Model file for the job. Use its own axes, mm. A direction names the side the tool comes from. Give positions to 0.01 mm unless a question says otherwise; leave off trailing zeros. Write each loop counter-clockwise with the first axis right and the second up, starting at its lowest first coordinate (ties: lowest second). Pieces come first, ordered by that corner, then holes.
```python
from build123d import *

# Parameters (mm, degrees)
SKIZZE1_R                       = 12.4
AUFSATZ_LINEAR_AUSTRAGEN1_DEPTH = 38.8
SKIZZE2_R                       = 3.75
AUFSATZ_LINEAR_AUSTRAGEN2_DEPTH = 2
SKIZZE3_R                       = 2
AUFSATZ_LINEAR_AUSTRAGEN3_DEPTH = 10
SKIZZE4_W                       = 7
SKIZZE4_H                       = 2
AUFSATZ_LINEAR_AUSTRAGEN4_DEPTH = 3


with BuildPart() as part:
    # Skizze1 → Aufsatz-Linear austragen1 (new body)
    with BuildSketch(Plane.XY):
        Circle(SKIZZE1_R)
    extrude(amount=AUFSATZ_LINEAR_AUSTRAGEN1_DEPTH)

    # Skizze2 → Aufsatz-Linear austragen2 (add)
    with BuildSketch(Plane.XY.offset(38.8)):
        Circle(SKIZZE2_R)
    extrude(amount=AUFSATZ_LINEAR_AUSTRAGEN2_DEPTH)

    # Skizze3 → Aufsatz-Linear austragen3 (add)
    with BuildSketch(Plane.XY.offset(40.8)):
        Circle(SKIZZE3_R)
    extrude(amount=AUFSATZ_LINEAR_AUSTRAGEN3_DEPTH)

    # Skizze4 → Aufsatz-Linear austragen4 (add)
    with BuildSketch(Plane(origin=(0, 0, 0), x_dir=(-1, 0, 0), z_dir=(0, 0, -1))):
        with Locations((0, -9)):
            Rectangle(SKIZZE4_W, SKIZZE4_H)
    extrude(amount=AUFSATZ_LINEAR_AUSTRAGEN4_DEPTH)


solid = part.part
```
1. Probe probe 1 along Z at (x, y) = (1.5, -10.5); probe 2 along Z at (x, y) = (-1.5, -2); probe 3 along X at (y, z) = (-0.25, 19). List the from-to ranges inside material, lowest first.
Calculated:
probe 1: z = 0 to 38.8
probe 2: z = 0 to 40.8
probe 3: x = -12.4 to 12.4
2. Pull direction Y, two halves, no side cores. Call faces 1 (the flat face through (0, -9, -3)), 2 (the flat face through (0, -8, -1)), 3 (the flat face through (0, -10, -1)), 4 (the cylindrical face through (0, -2, 46)): +Y half, -Y half, draft (parallel to the pull), parting line (faces both ways), or undercut.
Calculated:
face 1: draft
face 2: +Y half
face 3: -Y half
face 4: parting line
3. Slice it at C-C, the plane z = 30. Write the cut outline in (x, y).
Calculated:
outline: circle Ø24.8 at (0, 0)
4. Which spindle directions (+Z, -Z, +X, -X, +Y, -Y) get a long thin tool onto all of the face, cutting with end or side? Do faces 5 (the cylindrical face through (5.72, -11, 19.13)), 6 (the flat face through (2, -2, 40.8)), 7 (the flat face through (-3.5, -9, -1)), 8 (the flat face through (3.5, -9, -1)). Say none if no direction does.
Calculated:
face 5: +Z, -Z
face 6: +Z
face 7: -Z, -X, +Y, -Y
face 8: -Z, +X, +Y, -Y
5. Slice it at A-A, the plane x = 0. Write the cut outline in (y, z), and give its area (3 significant figures).
Calculated:
outline: (-12.4, 0) - (-10, 0) - (-10, -3) - (-8, -3) - (-8, 0) - (12.4, 0) - (12.4, 38.8) - (3.75, 38.8) - (3.75, 40.8) - (2, 40.8) - (2, 50.8) - (-2, 50.8) - (-2, 40.8) - (-3.75, 40.8) - (-3.75, 38.8) - (-12.4, 38.8) - close
area: 1,020 mm2
6. Slice it at B-B, the plane y = 0. Write the cut outline in (x, z), and give its area (3 significant figures).
Calculated:
outline: (-12.4, 0) - (12.4, 0) - (12.4, 38.8) - (3.75, 38.8) - (3.75, 40.8) - (2, 40.8) - (2, 50.8) - (-2, 50.8) - (-2, 40.8) - (-3.75, 40.8) - (-3.75, 38.8) - (-12.4, 38.8) - close
area: 1,020 mm2
7. Pin check, flat tips, straight feed: P1, Ø6, axis at y = -8.5, z = 26, coming from the +X side; P2, Ø4, axis at x = 8, y = 2, coming from the -Z side; P3, Ø1, axis at y = -8.5, z = -1, coming from the +X side. Stop position of each tip, or through.
Calculated:
P1: stops at x = 11.11
P2: stops at z = 0
P3: stops at x = 3.5
8. Slice it at D-D, the plane y = 9. Write the cut outline in (x, z).
Calculated:
outline: (-8.53, 0) - (8.53, 0) - (8.53, 38.8) - (-8.53, 38.8) - close
